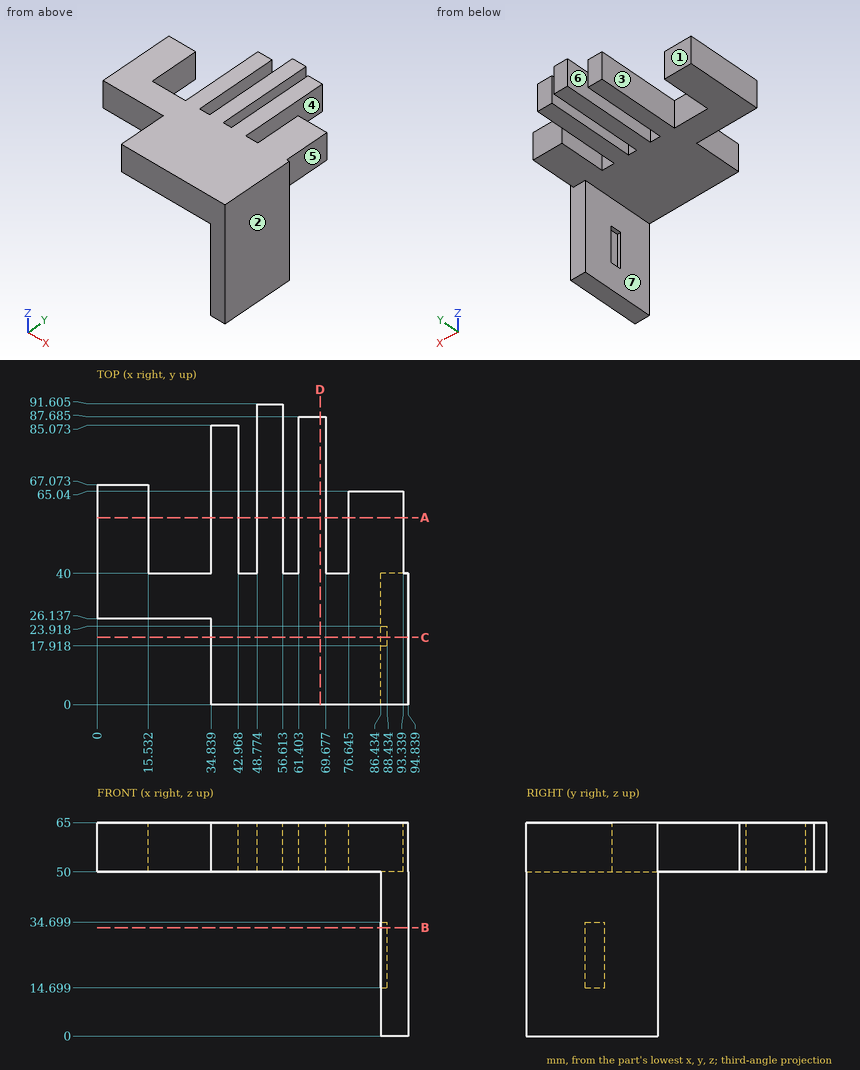
Verification items for this drawing (mm, ordinates from the low corner). A direction names the side the tool comes from. Give positions to 0.01 mm unless a question says otherwise; leave off trailing zeros. Loops run counter-clockwise (first coordinate to the right, second up) from the corner with the lowest first, then second, coordinate; pieces in that order, holes last. Notation, with made-up numbers: M 38.25,42 L 48.25,42 A35 cw 48.25,80 Z; hole C -11.75,59.5 d2. An arc over 180 degrees is marked long. Answer as CSV lines item,"result".
Item 1: Cross-section at D-D on x = 68. Record the cut outline in (y, z) (1 decimal).
Values:
outline,"M 0,50 L 87.7,50 L 87.7,65 L 0,65 Z"
Item 2: Depth check by flat-ended pin: P1, Ø4, axis at x = 65.5, z = 59.5, coming from the +Y side (1 decimal); P2, Ø2.5, axis at x = 39, z = 58.5, coming from the +Y side; P3, Ø1, axis at y = 62.5, z = 50.5, coming from the +X side; P4, Ø16.5, axis at y = 57.5, z = 54, coming from the -X side. Enter the tip coordinate at first touch or a pass-through.
Values:
P1,"stops at y = 87.7"
P2,"stops at y = 85.07"
P3,"stops at x = 93.34"
P4,"stops at x = 0"
Item 3: Release check for a two-part mould opening along X. For the marked faces 1, 2, 3 and 4 record: pulls with the +X half, pulls with the -X half, needs draft (parallel to the pull), parting line crosses it, or undercut.
Values:
face 1,"needs draft"
face 2,"pulls with the +X half"
face 3,"undercut"
face 4,"undercut"
Item 4: Material ranges on line 1 (Z direction, x = 87, y = 18); line 2 (Y direction, x = 88, z = 26.5); line 3 (Z direction, x = 78.5, y = 61), recorded low to high.
Values:
line 1,"z = 0 to 14.7, 34.7 to 65"
line 2,"y = 0 to 17.92, 23.92 to 40"
line 3,"z = 50 to 65"
Item 5: Cross-section at C-C on y = 20.5. Record the cut outline in (x, z) (1 decimal), and give its area (3 significant figures).
Values:
outline,"M 34.8,50 L 86.4,50 L 86.4,34.7 L 88.4,34.7 L 88.4,14.7 L 86.4,14.7 L 86.4,0 L 94.8,0 L 94.8,65 L 34.8,65 Z"
area,"1,280 mm²"
Item 6: Access from +Z, -Z, +X, -X, +Y, -Y to the whole of each face (thin tool, end or side, straight path). Record for the marked faces 5, 6 and 7.
Values:
face 5,"+Z, -Z, +X, +Y"
face 6,"+Z, -Z, +Y"
face 7,"-Z, -X, +Y, -Y"
Item 7: Cross-section at B-B on z = 33. Record the cut outline in (x, y) (1 decimal), and give its area (3 significant figures).
Values:
outline,"M 86.4,0 L 94.8,0 L 94.8,40 L 86.4,40 L 86.4,23.9 L 88.4,23.9 L 88.4,17.9 L 86.4,17.9 Z"
area,"324 mm²"
Item 8: Cross-section at A-A on y = 57. Record the cut outline in (x, z) (1 decimal).
Values:
outline,"M 0,50 L 15.5,50 L 15.5,65 L 0,65 Z; M 34.8,50 L 43,50 L 43,65 L 34.8,65 Z; M 48.8,50 L 56.6,50 L 56.6,65 L 48.8,65 Z; M 61.4,50 L 69.7,50 L 69.7,65 L 61.4,65 Z; M 76.6,50 L 93.3,50 L 93.3,65 L 76.6,65 Z"
